Input: part model. Units: mm. Frame: model coordinates. Face numbers are marked on the shaded views. Round coordinates to 2 decimals unless told otherwise and drop trailing zeros. Order: outer loops, then holes, each group sorted by start corner. A loop starts at its lowest first (then second) coordinate and runs counter-clockwise, first axis right, second up. Notation, with made-up numbers: M 32.25,-2.75 L 51.25,-2.75 A26 ccw 51.25,16.25 Z; hole C 41,22 d6. An arc over 180 degrees is marked long. One line per question, with ' | ' between items.
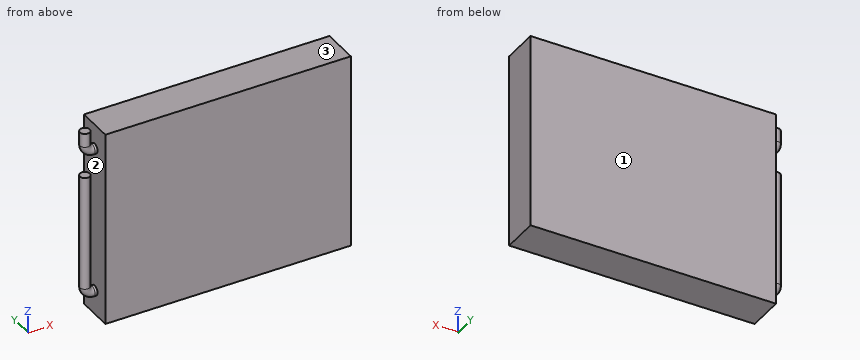
```python
from build123d import *

# Parameters (mm, degrees)
SKETCH1_W           = 50
SKETCH1_H           = 40.00000001
BOSS_EXTRUDE1_DEPTH = 7.5
SKETCH2_R           = 1
SKETCH4_R           = 1


with BuildPart() as part:
    # Sketch1 → Boss-Extrude1 (new body)
    with BuildSketch(Plane(origin=(0, 0, 0), x_dir=(1, 0, 0), z_dir=(0, 1, 0))):
        with Locations((25, 20.000000005)):
            Rectangle(SKETCH1_W, SKETCH1_H)
    extrude(amount=BOSS_EXTRUDE1_DEPTH)

    # Sweep1: sweep along a path in Sketch3
    with BuildLine(Plane(origin=(0, 3.75, 0), x_dir=(1, 0, 0), z_dir=(0, 1, 0))) as sweep1_path:
        Line((0, 35.000000005), (-0.5, 35.000000005))
        ThreePointArc((-0.5, 35.000000005), (-1.560660172, 34.560660177), (-2, 33.500000005))
        Line((-2, 33.500000005), (-2, 10.000000005))
    # Sketch2 → Sweep1 (sweep)
    with BuildSketch(Plane.ZY):
        with Locations((-35.000000005, 3.75)):
            Circle(SKETCH2_R)
    sweep(path=sweep1_path.line)

    # Sweep2: sweep along a path in Sketch5
    with BuildLine(Plane(origin=(0, 3.75, 0), x_dir=(1, 0, 0), z_dir=(0, 1, 0))) as sweep2_path:
        Line((0, 5), (-0.5, 5))
        ThreePointArc((-0.5, 5), (-1.560660172, 4.560660172), (-2, 3.5))
        Line((-2, 3.5), (-2, 0.674549329))
    # Sketch4 → Sweep2 (sweep)
    with BuildSketch(Plane.ZY):
        with Locations((-5, 3.75)):
            Circle(SKETCH4_R)
    sweep(path=sweep2_path.line)


solid = part.part
```
Item 1: Section query A-A, the plane z = -15. Return loops of the section in (x, y), plus the area to 3 significant figures.
Report:
outline: C -2,3.75 d2; M 0,0 L 50,0 L 50,7.5 L 0,7.5 Z | area: 378 mm²
Item 2: Section query B-B, the plane y = 3.75. Return loops of the section in (x, z), plus the area to 3 significant figures.
Report:
outline: M -3,-33.5 A2.5 ccw -0.5,-36 L 0,-36 L 0,-40 L 50,-40 L 50,0 L 0,0 L 0,-4 L -0.5,-4 A0.5 cw -1,-3.5 L -1,-0.67 L -3,-0.67 L -3,-3.5 A2.5 ccw -0.5,-6 L 0,-6 L 0,-34 L -0.5,-34 A0.5 cw -1,-33.5 L -1,-10 L -3,-10 Z | area: 2,060 mm²
Item 3: First-contact query: pin 1 (2 mm diameter, centred on x = -1.5, y = 3.5, fed in from +Z). Flat tip, straight axial feed; report the tip coordinate or a pass-through.
Report:
pin 1: z = -0.67
Item 4: Mould query, pull axis Z, two halves, no side actions, for the marked faces 1, 2 and 3. Classes: +Z half, -Z half, draft (parallel to the pull), parting line (faces both ways), or undercut.
Report:
face 1: draft | face 2: undercut | face 3: +Z half
Item 5: Line query: line 1 along X through (y, z) = (0.5, -30.5); line 2 along X through (y, z) = (4.5, -14); line 3 along X through (y, z) = (4.25, -23). Output: solid intervals per line, ascending. Write a range as from..to.
Report:
line 1: 0..50 | line 2: -2.66..-1.34, 0..50 | line 3: -2.87..-1.13, 0..50
